Read the model definition and answer for the solid it produces. Units are mm, in the model's axes. A direction names the side the tool comes from. Round coordinates to 2 decimals unless told otherwise and drop trailing zeros. Loops run counter-clockwise (first coordinate to the right, second up) from the corner with the lowest first, then second, coordinate; pieces in that order, holes last. Notation, with made-up numbers: M 86.5,-0.75 L 123.5,-0.75 A33 ccw 123.5,29.25 Z; hole C 77.5,3 d6. An arc over 180 degrees is marked long. Write each question's results on one line, items separated by ' | '.
```python
from build123d import *

# Parameters (mm, degrees)
BOSS_EXTRUDE1_DEPTH = 7.62
SKETCH2_R           = 33.285248113
SKETCH2_R_2         = 20.423872842
CUT_EXTRUDE1_DEPTH  = 6.0325
BOSS_EXTRUDE2_DEPTH = 2.54
BOSS_EXTRUDE3_DEPTH = 2.54
SKETCH5_W           = 4.7625
SKETCH5_H           = 6.35
BOSS_EXTRUDE4_DEPTH = 1.27
FILLET1_R           = 2.54
FILLET2_R           = 1.27


with BuildPart() as part:
    # Sketch1 → Boss-Extrude1 (new body)
    with BuildSketch(Plane(origin=(0, 0, 0), x_dir=(1, 0, 0), z_dir=(0, 1, 0))):
        with BuildLine():
            Line((0, 0), (25.4, 0))
            Line((25.4, 0), (25.4, 3.175))
            ThreePointArc((25.4, 3.175), (8.430498362, 8.430498362), (3.175, 25.4))
            Line((3.175, 25.4), (0, 25.4))
            Line((0, 25.4), (0, 0))
        make_face()
        with BuildLine():
            Line((2.54, 2.54), (2.54, 12.34659936))
            ThreePointArc((2.54, 12.34659936), (6.634447137, 6.634447137), (12.34659936, 2.54))
            Line((12.34659936, 2.54), (2.54, 2.54))
        make_face(mode=Mode.SUBTRACT)
    extrude(amount=BOSS_EXTRUDE1_DEPTH)

    # Sketch2 → Cut-Extrude1 (cut)
    with BuildSketch(Plane(origin=(0, 7.62, 0), x_dir=(1, 0, 0), z_dir=(0, 1, 0))):
        with Locations((21.900882543, 21.900882543)):
            Circle(SKETCH2_R)
        with Locations((21.900882543, 21.900882543)):
            Circle(SKETCH2_R_2, mode=Mode.SUBTRACT)
    extrude(amount=-CUT_EXTRUDE1_DEPTH, mode=Mode.SUBTRACT)

    # Sketch3 → Boss-Extrude2 (add)
    with BuildSketch(Plane.XY):
        Polygon((0, 0), (0, 6.35), (6.35, 6.35), (6.35, 1.5875), (19.05, 1.5875), (19.05, 6.35), (25.4, 6.35), (25.4, 0), align=None)
    extrude(amount=BOSS_EXTRUDE2_DEPTH)

    # Sketch4 → Boss-Extrude3 (add)
    with BuildSketch(Plane(origin=(0, 7.62, 0), x_dir=(1, 0, 0), z_dir=(0, 1, 0))):
        Polygon((3.175, 25.4), (0.889492523, 25.4), (0.889492523, 24.13), (2.981751079, 24.13), align=None)
        Polygon((25.4, 3.175), (25.4, 0.889492523), (24.13, 0.889492523), (24.13, 2.981751079), align=None)
    extrude(amount=BOSS_EXTRUDE3_DEPTH)

    # Sketch5 → Boss-Extrude4 (add)
    with BuildSketch(Plane(origin=(25.4, 0, 0), x_dir=(0, 0, -1), z_dir=(1, 0, 0))):
        with Locations((-2.38125, 3.175)):
            Rectangle(SKETCH5_W, SKETCH5_H)
    extrude(amount=BOSS_EXTRUDE4_DEPTH)

    # Fillet1
    # the kernel refuses this fillet: 2.54 mm, written as the material it adds along each edge
    with BuildSketch(Plane(origin=(19.05, 1.5875, 0), x_dir=(0, 1, 0), z_dir=(0, 0, 1))) as fillet1_piece_1:
        with BuildLine():
            CenterArc((FILLET1_R, FILLET1_R), FILLET1_R, 180, 90)
            Line((0, FILLET1_R), (0, 0))
            Line((0, 0), (FILLET1_R, 0))
        make_face()
    extrude(amount=2.54)
    with BuildSketch(Plane(origin=(6.35, 1.5875, 0), x_dir=(0, 1, 0), z_dir=(0, 0, 1))) as fillet1_piece_2:
        with BuildLine():
            CenterArc((FILLET1_R, -FILLET1_R), FILLET1_R, 90, 90)
            Line((0, -FILLET1_R), (0, 0))
            Line((0, 0), (FILLET1_R, 0))
        make_face()
    extrude(amount=2.54)
    with BuildSketch(Plane(origin=(-4.750979865, 7.62, -24.13), x_dir=(0, 0, 1), z_dir=(1, 0, 0))) as fillet1_piece_3_section:
        with BuildLine():
            CenterArc((FILLET1_R, -FILLET1_R), FILLET1_R, 90, 90)
            Line((0, -FILLET1_R), (0, 0))
            Line((0, 0), (FILLET1_R, 0))
        make_face()
    fillet1_piece_3 = extrude(amount=14.082730944, mode=Mode.PRIVATE)
    fillet1_piece_3 = fillet1_piece_3 & Plane(origin=(21.900882543, 8.195059905, -21.900882543), x_dir=(1, 0, 0), z_dir=(0, 1, 0)) * Cylinder(20.423872842, 39, mode=Mode.PRIVATE)
    fillet1_piece_3 = fillet1_piece_3 - Plane(origin=(21.900882543, 8.195059905, -21.900882543), x_dir=(0.18368070639060669, 0, 0.98298596027606), z_dir=(0, -1, 0)) * Cylinder(19.05, 39, mode=Mode.PRIVATE)
    add(fillet1_piece_3)
    with BuildSketch(Plane(origin=(24.13, 7.62, 4.750979865), x_dir=(0, 1, 0), z_dir=(0, 0, -1))) as fillet1_piece_4_section:
        with BuildLine():
            CenterArc((FILLET1_R, -FILLET1_R), FILLET1_R, 90, 90)
            Line((0, -FILLET1_R), (0, 0))
            Line((0, 0), (FILLET1_R, 0))
        make_face()
    fillet1_piece_4 = extrude(amount=14.082730944, mode=Mode.PRIVATE)
    fillet1_piece_4 = fillet1_piece_4 & Plane(origin=(21.900882543, 8.195056038, -21.900882543), x_dir=(1, 0, 0), z_dir=(0, 1, 0)) * Cylinder(20.423872842, 39, mode=Mode.PRIVATE)
    fillet1_piece_4 = fillet1_piece_4 - Plane(origin=(21.900882543, 8.195056038, -21.900882543), x_dir=(0.18368070639060669, 0, 0.98298596027606), z_dir=(0, -1, 0)) * Cylinder(19.05, 39, mode=Mode.PRIVATE)
    add(fillet1_piece_4)

    # Fillet2
    fillet2_edges = [part.edges().sort_by_distance(p)[0] for p in [
        (2.54, 0.79375, -12.34659936),
        (2.54, 0.79375, -2.54),
        (12.34659936, 0.79375, -2.54),
        (0, 0.79375, -25.4),
        (19.05, 6.35, 1.27),
        (6.35, 6.35, 1.27),
        (0, 6.35, 1.27),
        (0, 3.175, 2.54),
    ]]
    fillet(fillet2_edges, radius=FILLET2_R)


solid = part.part
```
1. Determine the mould class of faces 1 (the face through (19.412, 5.968, 1.288)), 2 (the face through (0.382, 0.805, -25.038)), 3 (the face through (23, 4, 0)), 4 (the face through (8, 1.588, -6)) for opening direction Z: released by +Z, released by -Z, zero draft, split by the parting line, or undercut.
Completed:
face 1: zero draft | face 2: released by -Z | face 3: undercut | face 4: undercut
2. Given P1, Ø0.6, axis at x = 24.5, y = 9, coming from the +Z side; P2, Ø6, axis at y = 5.5, z = -7, coming from the -X side; P3, Ø0.6, axis at y = 8.5, z = -1.5, coming from the -X side, each flat-ended and moving along its own axis, determine where each tip first touches the part or whether it passes through.
Completed:
P1: stops at z = -0.89 | P2: stops at x = 5.3 | P3: stops at x = 23.21
3. Find section B-B, the plane z = 0.5. Give the vertices of the cut face in (x, y), then the cut area to 3 significant figures.
Completed:
outline: M 0,0 L 26.67,0 L 26.67,6.35 L 20.32,6.35 A1.27 ccw 19.05,5.08 L 19.05,4.13 A2.54 cw 16.51,1.59 L 8.89,1.59 A2.54 cw 6.35,4.13 L 6.35,5.08 A1.27 ccw 5.08,6.35 L 1.27,6.35 A1.27 ccw 0,5.08 Z | area: 111 mm2
4. Find section C-C, the plane x = 7.5. Give the vertices of the cut face in (y, z).
Completed:
outline: M 0,-9.43 L 7.62,-9.43 L 7.62,-7.42 L 1.59,-7.42 L 1.59,-5.82 L 0,-5.82 Z; M 0,-2.54 L 1.59,-2.54 L 1.59,0 L 2,0 L 2,2.54 L 0,2.54 Z
5. Which of the six approach directions +Z, -Z, +X, -X, +Y, -Y give full straight-line access (tool end or side, diameter ignored) to faces 5 (the face through (9.135, 0.805, -3.421)), 6 (the face through (19.05, 4.6, 1.3)), 7 (the face through (25, 9, -0.889)), 8 (the face through (24.8, 7.62, -1.3)), 9 (the face through (3, 4, 0))?
Completed:
face 5: +Y, -Y | face 6: +Z, +Y | face 7: +Z, +X, -X, +Y | face 8: +Z, +X | face 9: +X, -X, +Y
6. Find the intervals of material crossed by L1, parallel to Z at x = 22.25, y = 5.75; L2, parallel to Y at x = 22, z = -1; L3, parallel to X at y = 5.5, z = 3, in increasing order.
Completed:
L1: z = -2.85 to -1.48, 0 to 2.54 | L2: y = 0 to 1.59 | L3: x = 25.4 to 26.67
7. Find section D-D, the plane y = 2.5. Count the separate pieces of the cut face and the enclosed holes in it, then the cut area to 3 significant figures.
Completed:
separate pieces: 3 | enclosed holes: 0 | area: 93.2 mm2
